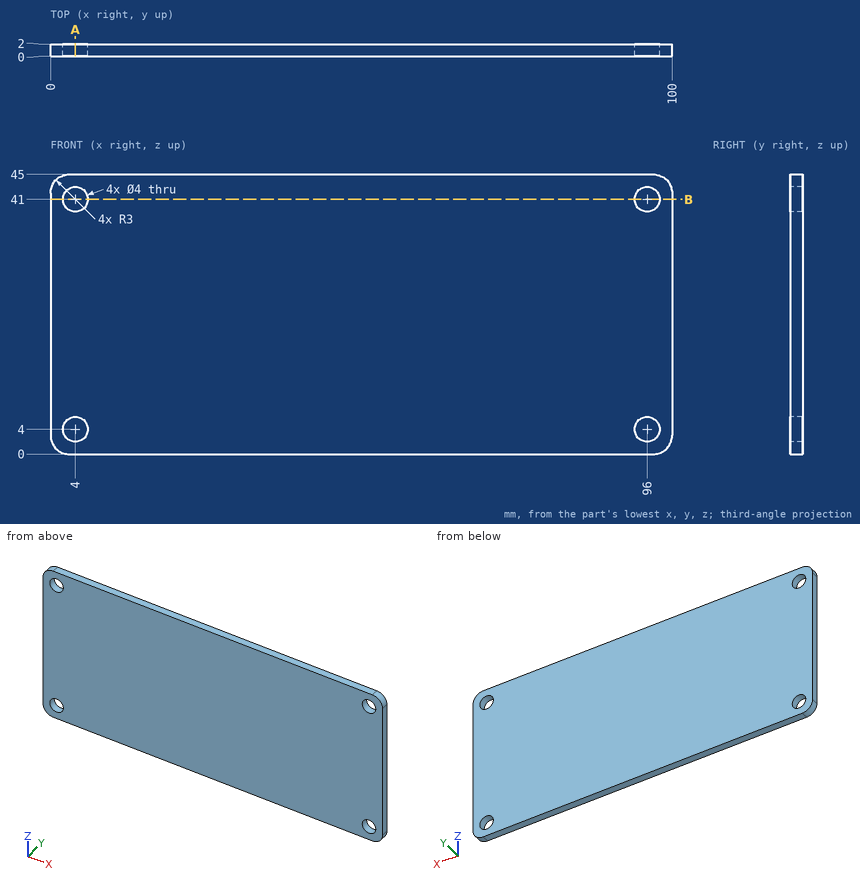
For this review, use the dimensioned drawing (mm, ordinates from the lowest corner) and the shaded views. Give positions to 0.01 mm unless a question says otherwise; leave off trailing zeros. Order: outer loops, then holes, each group sorted by start corner. A loop starts at its lowest first (then second) coordinate and runs counter-clockwise, first axis right, second up.
1) Insertion check: pin 1 (3.5 mm diameter, centred on x = 4, z = 4, fed in from -Y). The pin has a flat end and moves straight along its axis. Give the tip position at first contact, or say it passes through.
2) Take a section at B-B (z = 41). Give the boundary of the cut face in (x, y).
3) Wall thickness on line 1 (X direction, y = 1.4, z = 4); line 2 (Z direction, x = 96, y = 0.85); line 3 (X direction, y = 1.45, z = 3.5): over which ranges is each line inside the solid? List them lowest first.
4) Take a section at A-A (x = 4). Give the boundary of the cut face in (y, z), then the cut area to 3 significant figures.
Derived:
1. pin 1: passes through
2. outline: (0, 0) - (2, 0) - (2, 2) - (0, 2) - close; (6, 0) - (94, 0) - (94, 2) - (6, 2) - close; (98, 0) - (100, 0) - (100, 2) - (98, 2) - close
3. line 1: x = 0 to 2, 6 to 94, 98 to 100
3. line 2: z = 0 to 2, 6 to 39, 43 to 45
3. line 3: x = 0 to 2.06, 5.94 to 94.06, 97.94 to 100
4. outline: (0, 0) - (2, 0) - (2, 2) - (0, 2) - close; (0, 6) - (2, 6) - (2, 39) - (0, 39) - close; (0, 43) - (2, 43) - (2, 45) - (0, 45) - close
4. area: 74.0 mm2
